Autodesk Inventor part; units mm, degrees
ref_plane "IP1_XY" through (0, 0, 0) normal (1, 0, 0) x (0, 0, -1)
ref_plane "IP1_YZ" through (0, 0, 0) normal (0, 0, -1) x (0, 1, 0)
ref_plane "IP1_ZX" through (0, 0, 0) normal (0, 1, 0) x (1, 0, 0)
sketch "Sketch_1" plane through (0, 0, 0) normal (0, 1, 0) x (-1, 0, 0)
  line L0 (-10, 0) -> (6, 0)
  line L1 (0.4283, 0) -> (1.15, -1.25)
  line L2 (1.15, -1.25) -> (2.815, -1.25)
  line L3 (2.815, -1.25) -> (3, -1.435)
  line L4 (3, -1.435) -> (3, -2.45)
  arc A0 (2.7, -2.75) -> (3, -2.45) centre (2.7, -2.45) ccw
  line L5 (2.7, -2.75) -> (0, -2.75)
  line L6 (0, -2.75) -> (0, -1.8)
  arc A1 (0, -1.8) -> (-0.0562, -1.7101) centre (-0.1, -1.8) ccw
  line L7 (-0.0562, -1.7101) -> (-0.4662, -1.5101)
  arc A2 (-0.4662, -1.5101) -> (-0.51, -1.5) centre (-0.51, -1.6) ccw
  line L8 (-0.51, -1.5) -> (-9.6935, -1.5)
  line L9 (-9.6935, -1.5) -> (-10, -1.1935)
  line L10 (-10, -1.1935) -> (-10, 0)
  line L11 (-10, 0) -> (0.4283, 0)
revolve "Revolution1" add sketch "Sketch_1" angle 360 about axis through (10, 0, 0) along (1, 0, 0)
thread "Thread1"
sketch "Skizze_1" plane through (-1.15, 0, 0) normal (1, 0, 0) x (0, 0, -1)
  line L0 (-1.25, -0.7217) -> (0, -1.4434)
  line L1 (0, -1.4434) -> (1.25, -0.7217)
  line L2 (1.25, -0.7217) -> (1.25, 0.7217)
  line L3 (1.25, 0.7217) -> (0, 1.4434)
  line L4 (0, 1.4434) -> (-1.25, 0.7217)
  line L5 (-1.25, 0.7217) -> (-1.25, -0.7217)
extrude "Extrusion1" cut sketch "Skizze_1" against normal blind 2.6
ref_plane "IP1_XY" through (0, 0, 0) normal (1, 0, 0) x (0, 0, -1)
ref_plane "IP1_YZ" through (0, 0, 0) normal (0, 0, -1) x (0, 1, 0)
ref_plane "IP1_ZX" through (0, 0, 0) normal (0, 1, 0) x (1, 0, 0)
ref_plane "IP2_XY" through (-3, 0, 0) normal (1, 0, 0) x (0, 0, -1)
ref_plane "IP2_YZ" through (-3, 0, 0) normal (0, 0, -1) x (0, 1, 0)
ref_plane "IP2_ZX" through (-3, 0, 0) normal (0, 1, 0) x (1, 0, 0)
ref_plane "IP3_XY" through (10, 0, 0) normal (1, 0, 0) x (0, 0, -1)
ref_plane "IP3_YZ" through (10, 0, 0) normal (0, 0, -1) x (0, 1, 0)
ref_plane "IP3_ZX" through (10, 0, 0) normal (0, 1, 0) x (1, 0, 0)
ref_plane "IP4_XY" through (0, 0, 0) normal (1, 0, 0) x (0, 0, -1)
ref_plane "IP4_YZ" through (0, 0, 0) normal (0, 0, -1) x (0, 1, 0)
ref_plane "IP4_ZX" through (0, 0, 0) normal (0, 1, 0) x (1, 0, 0)
properties part number "Slotted head cap screw ISO 4762 - M3x10"
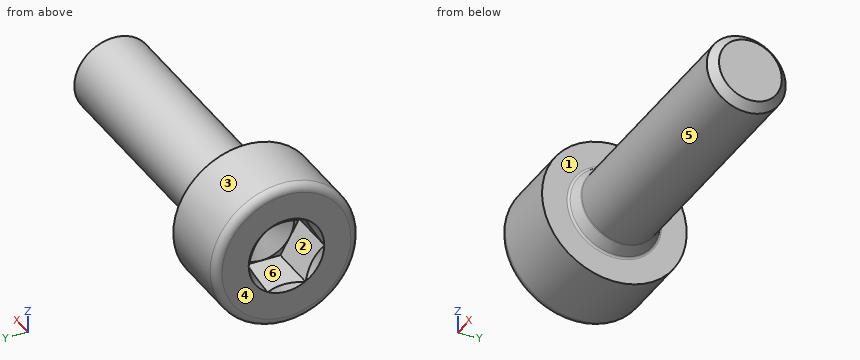
Model file for the job. Use its own axes, mm. Face numbers are marked on the shaded views. A direction names the side the tool comes from. Give positions to 0.01 mm unless a question says otherwise; leave off trailing zeros. Loops run counter-clockwise (first coordinate to the right, second up) from the corner with the lowest first, then second, coordinate; pieces in that order, holes last. Notation, with made-up numbers: (5.5, 85.25) -> (27.5, 85.25) arc R29 cw to (27.5, 112.25) -> close; hole circle Ø1 at (-17, -6.75). An arc over 180 degrees is marked (long way). Write each question's results on one line, items separated by ' | '.
(1) Pull direction Y, two halves, no side cores. Call the marked faces 4, 5 and 6: released by +Y, released by -Y, zero draft, split by the parting line, or undercut.
Geometry results:
face 4: zero draft | face 5: split by the parting line | face 6: undercut
(2) Cut at B-B on x = 3. List the corners of the cut face in (y, z).
Geometry results:
outline: circle Ø3 at (0, 0)
(3) Flat gauge pins, fed straight in: pin 1 Ø2 at (x, y) = (1.5, 2) entering from +Z; pin 2 Ø1 at (x, y) = (8.5, 0.5) entering from +Z; pin 3 Ø1 at (x, z) = (0, 1) entering from +Y. Where does each tip first touch, or does it go through?
Geometry results:
pin 1: stops at z = 1.12 | pin 2: stops at z = 1.5 | pin 3: stops at y = 2.7
(4) Cut at A-A on x = -0.75. List the corners of the cut face in (y, z), and give its area (3 significant figures).
Geometry results:
outline: circle Ø5.5 at (0, 0); hole circle Ø1.11 at (0, 0) | area: 22.8 mm²
(5) Tool access for the marked faces 1, 2 and 3: list every direction of +Z, -Z, +X, -X, +Y, -Y with a clear straight run to the whole face (end or side of a thin tool).
Geometry results:
face 1: +X | face 2: -X | face 3: +X, -X
(6) Probe line 1 along X through (y, z) = (-2.25, -0.05); line 2 along Z through (x, y) = (-1, -0.4); line 3 along Z through (x, y) = (3.5, 1.35). List the from-to ranges inside material, lowest first.
Geometry results:
line 1: x = -3 to 0 | line 2: z = -2.72 to -0.91, 0.91 to 2.72 | line 3: z = -0.65 to 0.65
